Source: three-view drawing plus pictorial views. Frame: mm from the lowest corner of the part. A direction names the side the tool comes from. Coordinates: 2 decimals unless noted, no trailing zeros. Order: outer loops, then holes, each group sorted by start corner. A loop starts at its lowest first (then second) coordinate and runs counter-clockwise, first axis right, second up. Notation, with made-up numbers: (54, 73.25) - (61, 73.25) arc R22 ccw to (61, 109.25) - close; hole circle Ø11 at (12.25, 81.5). An arc over 180 degrees is marked (long way). Use a Markdown table: item, result. Add a question column.
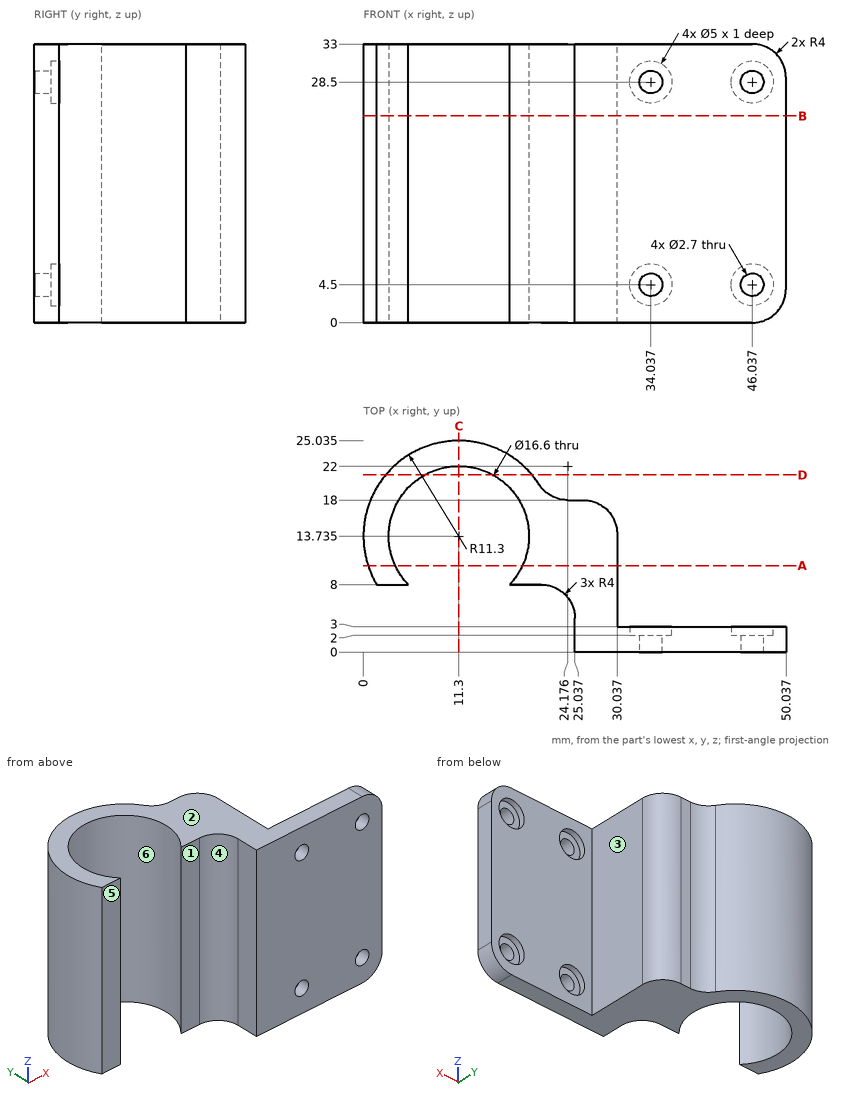
1) Draft query along X for the marked faces 4, 5 and 6. Return one class per face: pulls with the +X half, pulls with the -X half, needs draft (parallel to the pull), parting line crosses it, or undercut.
2) Set-up query: the marked faces 1, 2 and 3. Return all of +Z, -Z, +X, -X, +Y, -Y with unobstructed straight access to the full face (end or side cutting, diameter ignored); none if empty.
3) Section C-C (x = 11.3). Return loops of the section in (y, z) (1 decimal).
4) Section A-A (y = 10.25). Return loops of the section in (x, z).
5) Section B-B (z = 24.5). Return loops of the section in (x, y) (1 decimal).
6) Pin query (flat end, axial travel): pin 1 (3 mm diameter, centred on x = 18.5, z = 18.5, fed in from -Y); pin 2 (4 mm diameter, centred on x = 46.5, z = 3.5, fed in from +Y); pin 3 (3 mm diameter, centred on x = 34.04, z = 28.5, fed in from +Y); pin 4 (1.6 mm diameter, centred on x = 34.04, z = 28.5, fed in from -Y). Return the tip coordinate at first contact, or that it passes through.
7) Section D-D (y = 21). Return loops of the section in (x, z) (1 decimal).
8) Ray query, line 1 along X through (y, z) = (13.5, 27); line 2 along Y through (x, z) = (31.5, 23); line 3 along Y through (x, z) = (11.5, 15). Return the intervals inside material, ascending.
Values follow:
| question | item | result |
|---|---|---|
| 1 | face 4 | pulls with the -X half |
| 1 | face 5 | needs draft |
| 1 | face 6 | undercut |
| 2 | face 1 | +Z, -Z, -X, -Y |
| 2 | face 2 | +Z, +X, -X, +Y, -Y |
| 2 | face 3 | +Z, -Z, +X, +Y |
| 3 | outline | (22, 0) - (25, 0) - (25, 33) - (22, 33) - close |
| 4 | outline | (0.55, 0) - (3.77, 0) - (3.77, 33) - (0.55, 33) - close; (18.83, 0) - (30.04, 0) - (30.04, 33) - (18.83, 33) - close |
| 5 | outline | (1.6, 8) - (5.3, 8) arc R8.3 cw (long way) to (17.3, 8) - (21, 8) arc R4 cw to (25, 4) - (25, 0) - (50, 0) - (50, 3) - (30, 3) - (30, 14) arc R4 ccw to (26, 18) - (24.2, 18) arc R4 cw to (20.8, 19.8) arc R11.3 ccw to start |
| 6 | pin 1 | stops at y = 8 |
| 6 | pin 2 | stops at y = 3 |
| 6 | pin 3 | stops at y = 2 |
| 6 | pin 4 | passes through |
| 7 | outline | (2.6, 0) - (7.3, 0) - (7.3, 33) - (2.6, 33) - close; (15.3, 0) - (20, 0) - (20, 33) - (15.3, 33) - close |
| 8 | line 1 | x = 0 to 3, 19.6 to 30.04 |
| 8 | line 2 | y = 0 to 3 |
| 8 | line 3 | y = 22.03 to 25.03 |
